The listing builds one solid part. Answer for the finished solid, in the listing's coordinates (mm). A direction names the side the tool comes from. Round coordinates to 2 decimals unless told otherwise and drop trailing zeros. Order: outer loops, then holes, each group sorted by start corner. A loop starts at its lowest first (then second) coordinate and runs counter-clockwise, first axis right, second up. Notation, with made-up numbers: (22.25, 59.25) - (79.25, 59.25) arc R22 cw to (79.25, 94.25) - close; hole circle Ø3 at (14, 32.25). An arc over 180 degrees is marked (long way). Use CSV: the item, a comma, the result in double quotes. Start each with the question number.
Item 1: Find section B-B, the plane x = 0. Give the vertices of the cut face in (y, z), plus the area to 3 significant figures.
Item 2: Find section A-A, the plane z = 0. Give the vertices of the cut face in (x, y), plus the area to 3 significant figures.
Item 3: Straight lines are drawn through the part: line 1 along Y through (x, z) = (0.7, 1.1); line 2 along X through (y, z) = (4.25, -0.1); line 3 along Z through (x, y) = (0.45, 3.75). For each, find the intervals that lie inside material, in ascending order. Write a range as [from, to].
Item 4: Determine the mould class of faces 1 (the cylindrical face through (0, 3, 1)), 2 (the flat face through (0, -1, 0)), 3 (the flat face through (0, 6.5, 0)), 4 (the cylindrical face through (1.617, -0.394, -0.67)) for opening direction Y: +Y half, -Y half, draft (parallel to the pull), parting line (faces both ways), or undercut.
Item 5: For faces 5 (the flat face through (1, 0, -1)), 6 (the cylindrical face through (1.617, 5.894, 0.67)), determine the directions among +Z, -Z, +X, -X, +Y, -Y from which every point of the face is accessible in a straight line to the end or side of a thin tool.
Item 6: Find section C-C, the plane y = 2.25. Give the vertices of the cut face in (x, z), plus the area to 3 significant figures.
Item 7: A flat-ended cylindrical pin translates along its axis: P1, Ø1, axis at y = 1.5, z = -0.5, coming from the +X side. Find the tip coordinate at first contact, or state that the pin passes through.
```python
from build123d import *

# Parameters (mm, degrees)
SKETCH1_R           = 1
BOSS_EXTRUDE1_DEPTH = 5.5
SKETCH2_R           = 1.75
BOSS_EXTRUDE2_DEPTH = 1
CHAMFER1_SIZE       = 0.2
SKETCH3_R           = 1.75
BOSS_EXTRUDE3_DEPTH = 1
CHAMFER2_SIZE       = 0.2


with BuildPart() as part:
    # Sketch1 → Boss-Extrude1 (new body)
    with BuildSketch(Plane(origin=(0, 0, 0), x_dir=(1, 0, 0), z_dir=(0, 1, 0))):
        Circle(SKETCH1_R)
    extrude(amount=BOSS_EXTRUDE1_DEPTH)

    # Sketch2 → Boss-Extrude2 (add)
    with BuildSketch(Plane(origin=(0, 5.5, 0), x_dir=(1, 0, 0), z_dir=(0, 1, 0))):
        Circle(SKETCH2_R)
    extrude(amount=BOSS_EXTRUDE2_DEPTH)

    # Chamfer1
    chamfer1_edges = [part.edges().sort_by_distance(p)[0] for p in [
        (-1.75, 6.5, 0),
    ]]
    chamfer(chamfer1_edges, length=CHAMFER1_SIZE)

    # Sketch3 → Boss-Extrude3 (add)
    with BuildSketch(Plane.XZ):
        Circle(SKETCH3_R)
    extrude(amount=BOSS_EXTRUDE3_DEPTH)

    # Chamfer2
    chamfer2_edges = [part.edges().sort_by_distance(p)[0] for p in [
        (-1.75, -1, 0),
    ]]
    chamfer(chamfer2_edges, length=CHAMFER2_SIZE)


solid = part.part
```
Worked out:
1,outline,"(-1, -1.55) - (-0.8, -1.75) - (0, -1.75) - (0, -1) - (5.5, -1) - (5.5, -1.75) - (6.3, -1.75) - (6.5, -1.55) - (6.5, 1.55) - (6.3, 1.75) - (5.5, 1.75) - (5.5, 1) - (0, 1) - (0, 1.75) - (-0.8, 1.75) - (-1, 1.55) - close"
1,area,"17.9 mm²"
2,outline,"(-1.75, -0.8) - (-1.55, -1) - (1.55, -1) - (1.75, -0.8) - (1.75, 0) - (1, 0) - (1, 5.5) - (1.75, 5.5) - (1.75, 6.3) - (1.55, 6.5) - (-1.55, 6.5) - (-1.75, 6.3) - (-1.75, 5.5) - (-1, 5.5) - (-1, 0) - (-1.75, 0) - close"
2,area,"17.9 mm²"
3,line 1,"y = [-1, 0], [5.5, 6.5]"
3,line 2,"x = [-0.99, 0.99]"
3,line 3,"z = [-0.89, 0.89]"
4,face 1,"undercut"
4,face 2,"-Y half"
4,face 3,"+Y half"
4,face 4,"draft"
5,face 5,"none"
5,face 6,"+Y, -Y"
6,outline,"circle Ø2 at (0, 0)"
6,area,"3.14 mm²"
7,P1,"stops at x = 1"
